Verification items for the finished model (mm, model axes). Face numbers are marked on the shaded views. Coordinates: 2 decimals unless noted, no trailing zeros. Order: outer loops, then holes, each group sorted by start corner. A loop starts at its lowest first (then second) coordinate and runs counter-clockwise, first axis right, second up. Notation, with made-up numbers: M 71,72.25 L 80,72.25 A7 ccw 80,79.25 Z; hole C 28,72 d10. An arc over 180 degrees is marked long. Answer as a JSON object with one key per item and string values. Group by question number.
(1) Mould release check, pull along Z, two halves, no side actions. Record for the marked faces 1, 2, 3 and 4: released by +Z, released by -Z, zero draft, split by the parting line, or undercut.
(2) Cross-section at C-C (x = -4.5). Enter the section's corners in (y, z), plus the area to 3 significant figures.
(3) Cross-section at A-A (x = -10.5). Enter the section's corners in (y, z), plus the area to 3 significant figures.
(4) Cross-section at B-B (z = -1.5). Enter the section's corners in (x, y), plus the area to 3 significant figures.
(5) Gauge pin test, flat ends, axial feed: pin 1 Ø1.5 at (x, z) = (-7.5, 10.5) entering from -Y; pin 2 Ø4 at (x, z) = (-8.5, 8.5) entering from -Y; pin 3 Ø3.5 at (x, y) = (-3.5, -6.06) entering from -Z. Record the tip position at first contact, or that the pin passes through.
(6) Cross-section at D-D (x = 7). Count the separate pieces of the cut face and the enclosed holes in it, plus the area to 3 significant figures.
(7) Material ranges on line 1 (Y direction, x = -3.5, z = 7); line 2 (Y direction, x = 0.5, z = 2.5); line 3 (Z direction, x = 7.5, y = 13), recorded low to high.
from build123d import *
from build123d.topology import SkipClean

# Parameters (mm, degrees)
SKETCH1_R           = 18.5
BOSS_EXTRUDE1_DEPTH = 3
SKETCH2_R           = 11
BOSS_EXTRUDE2_DEPTH = 3.5
SKETCH4_R           = 3.05
CUT_EXTRUDE1_DEPTH  = 4.1
SKETCH5_R           = 1.5
CUT_EXTRUDE2_DEPTH  = 4
SKETCH7_R           = 11
SKETCH7_R_2         = 3
BOSS_EXTRUDE3_DEPTH = 11
SKETCH9_R           = 1.5
CUT_EXTRUDE4_DEPTH  = 32.476181471
SKETCH10_R          = 3
CUT_EXTRUDE5_DEPTH  = 32.476181471
SKETCH11_R          = 3.25
CUT_EXTRUDE8_DEPTH  = 10
BOSS_EXTRUDE4_START = 7
SKETCH12_R          = 18.5
SKETCH12_R_2        = 3.25
SKETCH12_R_3        = 3.05
BOSS_EXTRUDE4_DEPTH = 7
CUT_EXTRUDE9_START  = -5
SKETCH13_R          = 1.5
CUT_EXTRUDE9_DEPTH  = 17
CIRPATTERN1_COUNT   = 3


with BuildPart() as part:
    # Sketch1 → Boss-Extrude1 (new body)
    with BuildSketch(Plane.XY):
        Circle(SKETCH1_R)
    extrude(amount=BOSS_EXTRUDE1_DEPTH)

    # Sketch2 → Boss-Extrude2 (add)
    with BuildSketch(Plane.XY.offset(3)):
        Circle(SKETCH2_R)
    extrude(amount=BOSS_EXTRUDE2_DEPTH)

    # Sketch4 → Cut-Extrude1 (cut)
    with BuildSketch(Plane(origin=(0, 0, 0), x_dir=(-1, 0, 0), z_dir=(0, 0, -1))):
        Circle(SKETCH4_R)
    extrude(amount=-CUT_EXTRUDE1_DEPTH, mode=Mode.SUBTRACT)

    # Sketch5 → Cut-Extrude2 (cut)
    with BuildSketch(Plane(origin=(0, 0, 4.1), x_dir=(-1, 0, 0), z_dir=(0, 0, -1))):
        Circle(SKETCH5_R)
    extrude(amount=-CUT_EXTRUDE2_DEPTH, mode=Mode.SUBTRACT)

    # Sketch7 → Boss-Extrude3 (add)
    with BuildSketch(Plane.XY.offset(6.5)):
        Circle(SKETCH7_R)
        Circle(SKETCH7_R_2, mode=Mode.SUBTRACT)
    extrude(amount=BOSS_EXTRUDE3_DEPTH)

    # Sketch9 → Cut-Extrude4 (cut, through all)
    with BuildSketch(Plane.XY.offset(17.5)):
        with Locations((7, 0)):
            Circle(SKETCH9_R)
        with Locations((-3.5, -6.062177826)):
            Circle(SKETCH9_R)
        with Locations((-3.5, 6.062177826)):
            Circle(SKETCH9_R)
    extrude(amount=-CUT_EXTRUDE4_DEPTH, mode=Mode.SUBTRACT)

    # Sketch10 → Cut-Extrude5 (cut, through all)
    with SkipClean():  # the faces are left unmerged after this step: merging them gives an invalid solid
        with BuildSketch(Plane.XY.offset(17.5)):
            with Locations(Location((0, 0, 0), (0, 0, 180))):
                Circle(SKETCH10_R)
        extrude(amount=-CUT_EXTRUDE5_DEPTH, mode=Mode.SUBTRACT)

    # Sketch11 → Cut-Extrude8 (cut)
    with SkipClean():  # the faces are left unmerged after this step: merging them gives an invalid solid
        with BuildSketch(Plane(origin=(0, 0, 0), x_dir=(-1, 0, 0), z_dir=(0, 0, -1))):
            with Locations((3.5, -6.062177826)):
                Circle(SKETCH11_R)
            with Locations((3.5, 6.062177826)):
                Circle(SKETCH11_R)
            with Locations((-7, 0)):
                Circle(SKETCH11_R)
        extrude(amount=-CUT_EXTRUDE8_DEPTH, mode=Mode.SUBTRACT)
    add(part.part.scale(1), mode=Mode.REPLACE)  # the faces are merged on a copy

    # Sketch12 → Boss-Extrude4 (add)
    with BuildSketch(Plane(origin=(0, 0, 0), x_dir=(-1, 0, 0), z_dir=(0, 0, -1)).offset(BOSS_EXTRUDE4_START)):
        Circle(SKETCH12_R)
        with Locations((3.5, 6.062177826)):
            Circle(SKETCH12_R_2, mode=Mode.SUBTRACT)
        with Locations((3.5, -6.062177826)):
            Circle(SKETCH12_R_2, mode=Mode.SUBTRACT)
        with Locations((-7, 0)):
            Circle(SKETCH12_R_2, mode=Mode.SUBTRACT)
        Circle(SKETCH12_R_3, mode=Mode.SUBTRACT)
    extrude(amount=-BOSS_EXTRUDE4_DEPTH)

    # Sketch13 → Cut-Extrude9 (cut)
    with BuildSketch(Plane(origin=(0, 0, 0), x_dir=(0, 0, -1), z_dir=(1, 0, 0)).offset(CUT_EXTRUDE9_START)):
        with Locations((2, 0)):
            Circle(SKETCH13_R)
    cut_extrude9 = extrude(amount=-CUT_EXTRUDE9_DEPTH, mode=Mode.SUBTRACT)

    # CirPattern1: Cut-Extrude9 ×3 about axis
    cirpattern1_axis = Axis((0, 0, 0), (0, 0, 1))
    for i in range(1, CIRPATTERN1_COUNT):
        add(cut_extrude9.rotate(cirpattern1_axis, i * 360 / CIRPATTERN1_COUNT), mode=Mode.SUBTRACT)


solid = part.part
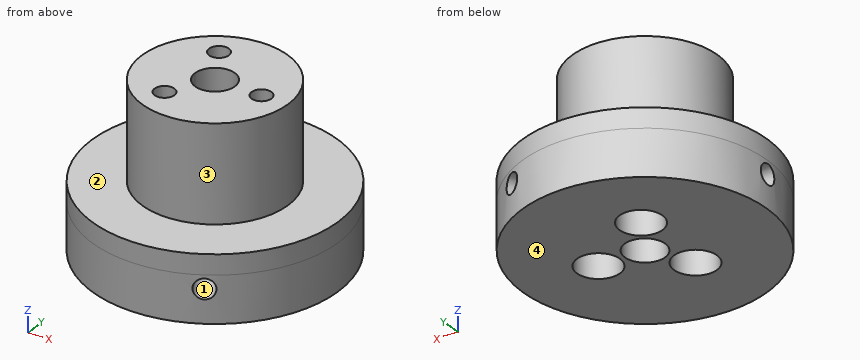
Taken from the geometry:
{
 "1": {"face 1": "undercut", "face 2": "released by +Z", "face 3": "zero draft", "face 4": "released by -Z"},
 "2": {"outline": "M -17.94,-7 L -9.15,-7 L -9.15,10 L -7.18,10 L -7.18,17.5 L -10.04,17.5 L -10.04,3 L -17.94,3 Z; M -4.94,10 L -2.97,10 L -2.97,-7 L 2.97,-7 L 2.97,10 L 4.94,10 L 4.94,17.5 L -4.94,17.5 Z; M 7.18,10 L 9.15,10 L 9.15,-7 L 17.94,-7 L 17.94,3 L 10.04,3 L 10.04,17.5 L 7.18,17.5 Z", "area": "406 mm²"},
 "3": {"outline": "M -15.23,-7 L 15.23,-7 L 15.23,3 L 3.28,3 L 3.28,17.5 L -3.28,17.5 L -3.28,3 L -15.23,3 Z; hole C 0,-2 d3", "area": "393 mm²"},
 "4": {"outline": "M -18.45,-1.41 A18.5 ccw 8,-16.68 L 1.28,-5.04 L 3.72,-3.62 L 10.45,-15.27 A18.5 ccw 10.45,15.27 L 3.72,3.62 L 1.28,5.04 L 8,16.68 A18.5 ccw -18.45,1.41 L -5,1.41 L -5,-1.41 Z; hole C -3.5,-6.06 d6.5; hole C -3.5,6.06 d6.5; hole C 0,0 d6.1; hole C 7,0 d6.5", "area": "832 mm²"},
 "5": {"pin 1": "stops at y = -8.69", "pin 2": "stops at y = -8.87", "pin 3": "stops at z = 10"},
 "6": {"separate pieces": "2", "enclosed holes": "2", "area": "427 mm²"},
 "7": {"line 1": "y = -10.43 to -9.31, -2.81 to 2.81, 9.31 to 10.43", "line 2": "y = -18.49 to -3.01, 3.01 to 18.49", "line 3": "z = -7 to -3.5, -0.5 to 3"}
}
